from build123d import *

# Parameters (mm, degrees)
SALIENTE_EXTRUIR1_DEPTH      = 5
SALIENTE_EXTRUIR1_DEPTH_BACK = 13
CROQUIS1_R                   = 2.5
SALIENTE_EXTRUIR2_DEPTH      = 6.5
SALIENTE_EXTRUIR2_DEPTH_BACK = 10
CORTAR_EXTRUIR2_REACH        = 83.059
CROQUIS4_R                   = 3.1
CROQUIS4_W                   = 30
CROQUIS4_H                   = 13
CORTAR_EXTRUIR3_DEPTH        = 10
CORTAR_EXTRUIR3_DEPTH_BACK   = 10
CROQUIS5_R                   = 5.5
SALIENTE_EXTRUIR3_REACH      = 83.059
CROQUIS6_W                   = 15
CROQUIS6_H                   = 4.684186211
REDONDEO1_R                  = 7


with BuildPart() as part:
    # Croquis1 → Saliente-Extruir1 (new, two sides: drawn at the far end of the back side and taken through both)
    with BuildSketch(Plane(origin=(0, 0, 0), x_dir=(1, 0, 0), z_dir=(0, 1, 0)).offset(-SALIENTE_EXTRUIR1_DEPTH_BACK)):
        Polygon((0, 0), (60, 0), (60, 30), (60, 52.93), (47.5, 52.93), (47.5, 30), (12.5, 30), (12.5, 52.93), (0, 52.93), (0, 30), align=None)
        with Locations(Location((10, 15, 0), (0, 0, 270))):
            Circle(CROQUIS1_R, mode=Mode.SUBTRACT)
        with Locations(Location((50, 15, 0), (0, 0, 270))):
            Circle(CROQUIS1_R, mode=Mode.SUBTRACT)
    extrude(amount=SALIENTE_EXTRUIR1_DEPTH + SALIENTE_EXTRUIR1_DEPTH_BACK)

    # Croquis2 → Saliente-Extruir2 (add, two sides: drawn at the far end of the back side and taken through both)
    with BuildSketch(Plane(origin=(0, 5, 0), x_dir=(1, 0, 0), z_dir=(0, 1, 0)).offset(-SALIENTE_EXTRUIR2_DEPTH_BACK)):
        Polygon((3, 0), (3, 25), (17, 25), (17, 0), (43, 0), (43, 25), (57, 25), (57, 0), (60, 0), (60, 52.93), (47.5, 52.93), (47.5, 30), (12.5, 30), (12.5, 52.93), (0, 52.93), (0, 0), align=None)
    extrude(amount=SALIENTE_EXTRUIR2_DEPTH + SALIENTE_EXTRUIR2_DEPTH_BACK)

    # Cortar-Extruir2: up to this face of the body (flat: up to its plane)
    cortar_extruir2_end = Plane(part.part.faces().sort_by_distance((60, -0.75, -26.465))[0])
    # Croquis4 → Cortar-Extruir2 (cut, up to the picked face)
    with BuildSketch(Plane.ZY, mode=Mode.PRIVATE) as cortar_extruir2_sk1:
        with Locations((-43.93, -5.75)):
            Circle(CROQUIS4_R)
    cortar_extruir2_tool1 = split(extrude(cortar_extruir2_sk1.sketch, amount=-CORTAR_EXTRUIR2_REACH, mode=Mode.PRIVATE), bisect_by=cortar_extruir2_end, keep=Keep.BOTH, mode=Mode.PRIVATE)
    # Croquis4 → Cortar-Extruir2 (cut, up to the picked face)
    with BuildSketch(Plane.ZY, mode=Mode.PRIVATE) as cortar_extruir2_sk2:
        with Locations((-15, -6.5)):
            Rectangle(CROQUIS4_W, CROQUIS4_H)
    cortar_extruir2_tool2 = split(extrude(cortar_extruir2_sk2.sketch, amount=-CORTAR_EXTRUIR2_REACH, mode=Mode.PRIVATE), bisect_by=cortar_extruir2_end, keep=Keep.BOTH, mode=Mode.PRIVATE)
    add(cortar_extruir2_tool1.solids().sort_by(Axis((0, -5.75, -43.93), (1, 0, 0)))[0], mode=Mode.SUBTRACT)
    add(cortar_extruir2_tool2.solids().sort_by(Axis((0, -6.5, -15), (1, 0, 0)))[0], mode=Mode.SUBTRACT)

    # Croquis5 → Cortar-Extruir3 (cut, two sides: drawn at the far end of the back side and taken through both)
    with BuildSketch(Plane(origin=(0, -9.25, -9.25), x_dir=(-1, 0, 0), z_dir=(0, -0.7071067811865488, -0.7071067811865464)).offset(-CORTAR_EXTRUIR3_DEPTH_BACK)):
        with Locations((-30, 29.344931419)):
            Circle(CROQUIS5_R)
    extrude(amount=CORTAR_EXTRUIR3_DEPTH + CORTAR_EXTRUIR3_DEPTH_BACK, mode=Mode.SUBTRACT)

    # Saliente-Extruir3: up to this face of the body (flat: up to its plane)
    saliente_extruir3_end = Plane(part.part.faces().sort_by_distance((60, 1.98040053, -30.964309834))[0])
    # Croquis6 → Saliente-Extruir3 (add, up to the picked face)
    with BuildSketch(Plane.ZY, mode=Mode.PRIVATE) as saliente_extruir3_sk1:
        with Locations((-22.5, -10.657906894)):
            Rectangle(CROQUIS6_W, CROQUIS6_H)
    saliente_extruir3_tool1 = split(extrude(saliente_extruir3_sk1.sketch, amount=-SALIENTE_EXTRUIR3_REACH, mode=Mode.PRIVATE), bisect_by=saliente_extruir3_end, keep=Keep.BOTH, mode=Mode.PRIVATE)
    add(saliente_extruir3_tool1.solids().sort_by(Axis((0, -10.657907, -22.5), (1, 0, 0)))[0])

    # Redondeo1
    # the kernel refuses this fillet: 7 mm, written as the material it takes off along each edge
    with BuildSketch(Plane(origin=(-16.514578123, -13, -15), x_dir=(0, 0, -1), z_dir=(1, 0, 0))) as redondeo1_piece_1:
        with BuildLine():
            CenterArc((6.605831249, 7), REDONDEO1_R, 199.319193713, 70.680806287)
            Line((0, 4.684186211), (0, 0))
            Line((0, 0), (6.605831249, 0))
        make_face()
    extrude(amount=93.029156246, mode=Mode.SUBTRACT)
    with BuildSketch(Plane(origin=(77.5, -13, -52.93), x_dir=(0, 1, 0), z_dir=(-1, 0, 0)), Plane(origin=(30, 11.5, -52.93), x_dir=(0, 0, 1), z_dir=(-1, 0, 0)), Plane(origin=(77.5, 11.5, -52.93), x_dir=(0, 0, 1), z_dir=(-1, 0, 0))) as redondeo1_piece_2:
        with BuildLine():
            CenterArc((REDONDEO1_R, -REDONDEO1_R), REDONDEO1_R, 90, 90)
            Line((0, -REDONDEO1_R), (0, 0))
            Line((0, 0), (REDONDEO1_R, 0))
        make_face()
    extrude(amount=47.5, mode=Mode.SUBTRACT)
    with BuildSketch(Plane(origin=(30, -13, -52.93), x_dir=(0, 0, 1), z_dir=(-1, 0, 0))) as redondeo1_piece_3:
        with BuildLine():
            CenterArc((REDONDEO1_R, REDONDEO1_R), REDONDEO1_R, 180, 90)
            Line((0, REDONDEO1_R), (0, 0))
            Line((0, 0), (REDONDEO1_R, 0))
        make_face()
    extrude(amount=47.5, mode=Mode.SUBTRACT)
    with BuildSketch(Plane(origin=(-17.5, 11.5, 0), x_dir=(0, -1, 0), z_dir=(1, 0, 0)), Plane(origin=(39.5, 11.5, 0), x_dir=(0, -1, 0), z_dir=(1, 0, 0))) as redondeo1_piece_4:
        with BuildLine():
            CenterArc((REDONDEO1_R, REDONDEO1_R), REDONDEO1_R, 180, 90)
            Line((0, REDONDEO1_R), (0, 0))
            Line((0, 0), (REDONDEO1_R, 0))
        make_face()
    extrude(amount=38, mode=Mode.SUBTRACT)
    with BuildSketch(Plane(origin=(-0.5, 11.5, 0), x_dir=(0, -1, 0), z_dir=(1, 0, 0))) as redondeo1_piece_5:
        with BuildLine():
            CenterArc((REDONDEO1_R, REDONDEO1_R), REDONDEO1_R, 180, 90)
            Line((0, REDONDEO1_R), (0, 0))
            Line((0, 0), (REDONDEO1_R, 0))
        make_face()
    extrude(amount=61, mode=Mode.SUBTRACT)


solid = part.part
Design review of the part built by this model. Coordinates are the model's own, in mm. A direction names the side the tool comes from. Round coordinates to 2 decimals unless told otherwise and drop trailing zeros. Write each loop counter-clockwise with the first axis right and the second up, starting at its lowest first coordinate (ties: lowest second). Pieces come first, ordered by that corner, then holes. Notation, with made-up numbers: (2.5, 80.5) - (12.5, 80.5) arc R11 ccw to (12.5, 89.5) - close; hole circle Ø8 at (23.5, 77.5). An arc over 180 degrees is marked (long way). Return JSON: item names as keys, results as strings. Group by question number.
Item 1: We need section B-B on z = -40. Write out the cut boundary in (x, y), and give its area (4 significant figures).
Item 2: We need section A-A on x = 10. Write out the cut boundary in (y, z), and give its area (3 significant figures).
Item 3: For probe 1 along X at (y, z) = (3.75, -15); probe 2 along X at (y, z) = (-0.5, -42); probe 3 along Y at (x, z) = (58, -25), list the stretches that pass through material, from the lowest coordinate up. Write a range as [from, to].
Item 4: Insertion check: P1, Ø3, axis at x = 10, z = -15, coming from the +Y side; P2, Ø3, axis at x = 51, z = -14.5, coming from the +Y side; P3, Ø4, axis at x = 4, y = -5, coming from the +Z side. Each pin has a flat end and moves straight along its axis. Give the tip position at first contact, or say it passes through.
Item 5: We need section D-D on x = 31. Write out the cut boundary in (y, z), and give its area (3 significant figures).
Item 6: The part is to be moulded in two halves that separate along Y. For faces 6 (the face through (11.5, 5, -12.7)), 7 (the face through (60, 2, -32)), 8 (the face through (6.162, -6.937, -41.066)), say which applies: pulls with the +Y half, pulls with the -Y half, needs draft (parallel to the pull), parting line crosses it, or undercut.
Item 7: Machinability: for faces 1 (the face through (57, 8, -13)), 2 (the face through (30, -8.316, -23)), 3 (the face through (29.6, 9.5, -2.1)), 4 (the face through (12.5, -1, -41)), 5 (the face through (8.5, 2.5, -17)), which of the approach directions +Z, -Z, +X, -X, +Y, -Y give a long, thin tool a straight path to every point of the face, cutting with its end or side? Answer none if there is none.
Item 8: We need section C-C on x = 55. Write out the cut boundary in (y, z), and give its area (3 significant figures).
Model answer:
{
 "1": {"outline": "(0, -13) - (12.5, -13) - (12.5, 11.5) - (0, 11.5) - close; (47.5, -13) - (60, -13) - (60, 11.5) - (47.5, 11.5) - close", "area": "612.5 mm²"},
 "2": {"outline": "(-13, -45.93) arc R7 ccw to (-6, -52.93) - (4.5, -52.93) arc R7 ccw to (11.5, -45.93) - (11.5, -25) - (5, -25) - (5, -17.5) - (0, -17.5) - (0, -30) - (-8.32, -30) - (-8.32, -15) arc R7 ccw to (-13, -21.61) - close; (0, -12.5) - (5, -12.5) - (5, -0.02) arc R7 ccw to (4.5, 0) - (0, 0) - close; hole circle Ø6.2 at (-5.75, -43.93)", "area": "730 mm²"},
 "3": {"probe 1": "x = [0, 7.5], [12.5, 47.5], [52.5, 60]", "probe 2": "x = [0, 12.5], [47.5, 60]", "probe 3": "y = [-13, -8.32], [0, 11.5]"},
 "4": {"P1": "stops at y = -8.32", "P2": "stops at y = 5", "P3": "stops at z = -30"},
 "5": {"outline": "(-13, -30) - (-8.32, -30) - (-8.32, -15) arc R7 ccw to (-13, -21.61) - close; (0, -30) - (3.85, -30) - (11.5, -22.35) - (11.5, -7) arc R7 ccw to (4.5, 0) - (0, 0) - close", "area": "367 mm²"},
 "6": {"face 6": "pulls with the +Y half", "face 7": "needs draft", "face 8": "undercut"},
 "7": {"face 1": "+Z, +Y", "face 2": "+Z, +X, -X", "face 3": "+Z, +X, -X, +Y", "face 4": "-Z, +Y, -Y", "face 5": "+Y"},
 "8": {"outline": "(-13, -45.93) arc R7 ccw to (-6, -52.93) - (4.5, -52.93) arc R7 ccw to (11.5, -45.93) - (11.5, -25) - (5, -25) - (5, -0.02) arc R7 ccw to (4.5, 0) - (0, 0) - (0, -30) - (-8.32, -30) - (-8.32, -15) arc R7 ccw to (-13, -21.61) - close; hole circle Ø6.2 at (-5.75, -43.93)", "area": "755 mm²"}
}
